Job drawing, mm, ordinate dimensions from the low corner. One solid piece. A direction names the side the tool comes from. Coordinates: 2 decimals unless noted, no trailing zeros. Order: outer loops, then holes, each group sorted by start corner. A loop starts at its lowest first (then second) coordinate and runs counter-clockwise, first axis right, second up. Notation, with made-up numbers: (0, -1.75) - (18, -1.75) arc R29 ccw to (18, 21.25) - close; hole circle Ø4 at (75.25, -1). An arc over 180 degrees is marked (long way). Use a Markdown table: item, result. Add a question column.
1) Saw through at D-D on x = 0.6. List the corners of the cut face in (y, z).
2) Wall check: L1, parallel to Y at x = 3, z = 6; L2, parallel to Z at x = 1.2, y = 1.7. Give the ranges that are in metal, low to high. Write a range as [from, to].
3) Drop flat-ended pins along their axis: P1, Ø1.4, axis at x = 3, y = 3, coming from the -Z side; P2, Ø1, axis at x = 1, y = 2.5, coming from the -Z side. Give the stop position or say it passes through.
4) Saw through at A-A on y = 3. List the corners of the cut face in (x, z).
5) Two-plate mould, pull along X, no slides. Class the marked faces 1, 2 and 3: +X half, -X half, draft (parallel to the pull), parting line (faces both ways), or undercut.
6) Tool access for the marked faces 4 and 5: list every direction of +Z, -Z, +X, -X, +Y, -Y with a clear straight run to the whole face (end or side of a thin tool).
7) Saw through at C-C on z = 2.5. List the corners of the cut face in (x, y), then the cut area to 3 significant figures.
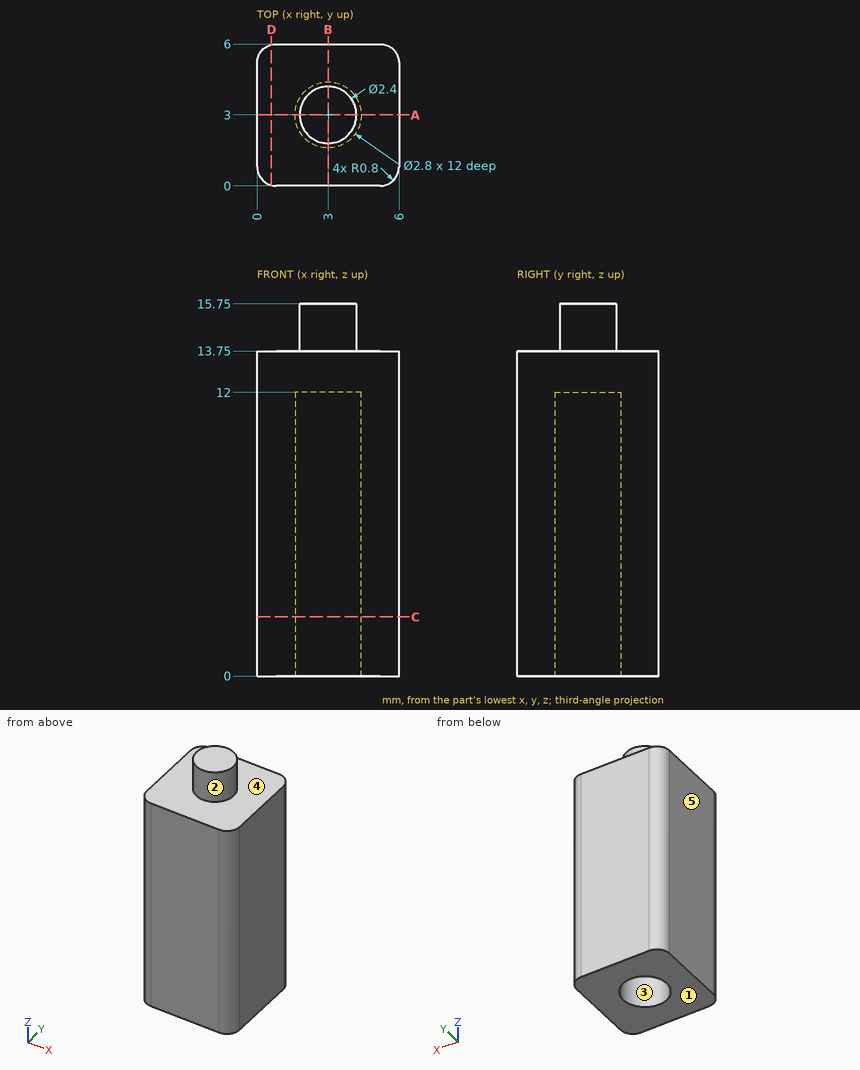
Results are:
| question | item | result |
|---|---|---|
| 1 | outline | (0.03, 0) - (5.97, 0) - (5.97, 13.75) - (0.03, 13.75) - close |
| 2 | L1 | [0, 1.6], [4.4, 6] |
| 2 | L2 | [0, 13.75] |
| 3 | P1 | z = 12 |
| 3 | P2 | z = 0 |
| 4 | outline | (0, 0) - (1.6, 0) - (1.6, 12) - (4.4, 12) - (4.4, 0) - (6, 0) - (6, 13.75) - (4.2, 13.75) - (4.2, 15.75) - (1.8, 15.75) - (1.8, 13.75) - (0, 13.75) - close |
| 5 | face 1 | draft |
| 5 | face 2 | parting line |
| 5 | face 3 | undercut |
| 6 | face 4 | +Z |
| 6 | face 5 | +Z, -Z, -X, +Y, -Y |
| 7 | outline | (0, 0.8) arc R0.8 ccw to (0.8, 0) - (5.2, 0) arc R0.8 ccw to (6, 0.8) - (6, 5.2) arc R0.8 ccw to (5.2, 6) - (0.8, 6) arc R0.8 ccw to (0, 5.2) - close; hole circle Ø2.8 at (3, 3) |
| 7 | area | 29.3 mm2 |
